```python
from build123d import *

# Parameters (mm, degrees)
SKETCH_1_R      = 1.6
EXTRUDE_1_DEPTH = 4
FILLET_1_R      = 3
FILLET_2_R      = 1


with BuildPart() as part:
    # ｽｹｯﾁ1 → ﾎﾞｽ - 押し出し1 (new body)
    with BuildSketch(Plane(origin=(0, 0, 0), x_dir=(1, 0, 0), z_dir=(0, 1, 0))):
        Polygon((-15, -4), (0, -4), (15, -4), (15, 0), (28, 0), (28, 13), (0, 13), (-23.545815275, 0), (-15, 0), align=None)
        with Locations((8, 8)):
            Circle(SKETCH_1_R, mode=Mode.SUBTRACT)
        with Locations((24, 8)):
            Circle(SKETCH_1_R, mode=Mode.SUBTRACT)
    extrude(amount=EXTRUDE_1_DEPTH)

    # ﾌｨﾚｯﾄ1
    fillet_1_edges = [part.edges().sort_by_distance(p)[0] for p in [
        (0, 2, -13),
        (28, 2, -13),
        (28, 2, 0),
    ]]
    fillet(fillet_1_edges, radius=FILLET_1_R)

    # ﾌｨﾚｯﾄ2
    fillet_2_edges = [part.edges().sort_by_distance(p)[0] for p in [
        (-23.545815275, 2, 0),
    ]]
    fillet(fillet_2_edges, radius=FILLET_2_R)


solid = part.part
```
The listing builds one solid part. Answer for the finished solid, in the listing's coordinates (mm). A direction names the side the tool comes from. Coordinates: 2 decimals unless noted, no trailing zeros. Loops run counter-clockwise (first coordinate to the right, second up) from the corner with the lowest first, then second, coordinate; pieces in that order, holes last. Notation, with made-up numbers: (31, 0.5) -> (84, 0.5) arc R25 cw to (84, 21.5) -> close; hole circle Ø8 at (55.25, 30). An arc over 180 degrees is marked (long way). Return JSON: item names as keys, results as strings. Group by question number.
(1) Given pin 1 Ø2 at (y, z) = (2, 1.5) entering from -X; pin 2 Ø1.2 at (x, y) = (-17.5, 2.5) entering from +Z; pin 3 Ø2 at (y, z) = (2.5, 2.5) entering from +X, each flat-ended and moving along its own axis, determine where each tip first touches the part or whether it passes through.
(2) Find the intervals of material crossed by probe 1 along X at (y, z) = (2.1, -8); probe 2 along X at (y, z) = (0.65, -7.25); probe 3 along Z at (x, y) = (24, 1.9), in increasing order. Write a range as from..to.
(3) A cutting plane is placed at B-B on z = -8. Write down the section's boundary in (x, y).
(4) A cutting plane is placed at D-D on x = 24. Write down the section's boundary in (y, z), and give its area (3 significant figures).
(5) A cutting plane is placed at A-A on x = 8. Write down the section's boundary in (y, z).
(6) Which of the six approach directions +Z, -Z, +X, -X, +Y, -Y give full straight-line access (tool end or side, diameter ignored) to faces 1 (the flat face through (28, 2, -6)), 2 (the flat face through (20, 2, 0)), 3 (the flat face through (-17, 2, 0))?
(7) A cutting plane is placed at C-C on y = 0.5. Write down the section's boundary in (x, z).
(8) Determine the mould class of faces 4 (the cylindrical face through (-20.63, 2.03, -0.73)), 5 (the flat face through (3, 0, -5)), 6 (the flat face through (15, 2, 2)), 7 (the cylindrical face through (6.73, 1.97, -7.03)) for opening direction X: released by +X, released by -X, zero draft, split by the parting line, or undercut.
The answers:
{
 "1": {"pin 1": "stops at x = -15", "pin 2": "stops at z = 0", "pin 3": "stops at x = 15"},
 "2": {"probe 1": "x = -9.06..6.4, 9.6..22.4, 25.6..28", "probe 2": "x = -10.41..6.59, 9.41..22.59, 25.41..28", "probe 3": "z = -13..-9.6, -6.4..0"},
 "3": {"outline": "(-9.06, 0) -> (6.4, 0) -> (6.4, 4) -> (-9.06, 4) -> close; (9.6, 0) -> (22.4, 0) -> (22.4, 4) -> (9.6, 4) -> close; (25.6, 0) -> (28, 0) -> (28, 4) -> (25.6, 4) -> close"},
 "4": {"outline": "(0, -13) -> (4, -13) -> (4, -9.6) -> (0, -9.6) -> close; (0, -6.4) -> (4, -6.4) -> (4, 0) -> (0, 0) -> close", "area": "39.2 mm^2"},
 "5": {"outline": "(0, -13) -> (4, -13) -> (4, -9.6) -> (0, -9.6) -> close; (0, -6.4) -> (4, -6.4) -> (4, 4) -> (0, 4) -> close"},
 "6": {"face 1": "+Z, -Z, +X, +Y, -Y", "face 2": "+Z, +X, +Y, -Y", "face 3": "+Z, -X, +Y, -Y"},
 "7": {"outline": "(-20.15, -1.88) -> (-0.68, -12.63) arc R3 ccw to (0.77, -13) -> (25, -13) arc R3 ccw to (28, -10) -> (28, -3) arc R3 ccw to (25, 0) -> (15, 0) -> (15, 4) -> (-15, 4) -> (-15, 0) -> (-19.67, 0) arc R1 ccw to start; hole circle Ø3.2 at (8, -8); hole circle Ø3.2 at (24, -8)"},
 "8": {"face 4": "released by -X", "face 5": "zero draft", "face 6": "released by +X", "face 7": "undercut"}
}
